CAD build for the part. Positions are in the model's coordinates, mm. A direction names the side the tool comes from. Coordinates: 2 decimals unless noted, no trailing zeros. Write each loop counter-clockwise with the first axis right and the second up, starting at its lowest first coordinate (ties: lowest second). Pieces come first, ordered by that corner, then holes. Notation, with made-up numbers: (-23, 41.25) - (25, 41.25) arc R26 ccw to (25, 61.25) - close; hole circle Ø6 at (79.25, -37.5). An arc over 180 degrees is marked (long way). One line per question, with ' | ' between items. Start each with the question number.
1. Band-saw the part on A-A, the plane z = -101. Write the cut outline in (x, y).
2. Two-plate mould, pull along X, no slides. Class faces 1 (the cylindrical face through (7.587, 34.168, 9.479)), 2 (the cylindrical face through (-28.4, -28.36, -60.49)), 3 (the cylindrical face through (-29.2, 29.81, 3.94)): +X half, -X half, draft (parallel to the pull), parting line (faces both ways), or undercut.
3. Band-saw the part on C-C, the plane y = -20.5. Write the cut outline in (x, z).
4. Flat gauge pins, fed straight in: P1, Ø8.5, axis at x = 31.82, y = 31.82, coming from the -Z side; P2, Ø7, axis at x = -35, z = -36, coming from the -Y side; P3, Ø2.5, axis at y = -33, z = -32, coming from the +X side; P4, Ø5.5, axis at x = 1, y = -0.5, coming from the +Z side. Where does each tip first touch, or does it go through?
5. Band-saw the part on B-B, the plane x = 0. Write the cut outline in (y, z).
6. Probe line 1 (Y direction, x = 0, z = 40); line 2 (Z direction, x = -12, y = -2); line 3 (Y direction, x = 31.5, z = -48.5). List the from-to ranges inside material, lowest first.
7. Band-saw the part on D-D, the plane x = -23. Write the cut outline in (y, z).
8. Which spindle directions (+Z, -Z, +X, -X, +Y, -Y) get a long thin tool onto all of the face, cutting with end or side? Do faces 4 (the flat face through (27.5, 35, -59)), 5 (the cylindrical face through (-28.4, 28.36, -60.49)), 6 (the flat face through (-35, -35, 0)), 7 (the flat face through (0, 12, 31)), 8 (the flat face through (0, 0, 33)). Say none if no direction does.
from build123d import *

# Parameters (mm, degrees)
SKETCH_1_W              = 80
SKETCH_1_H              = 80
EXTRUDE_1_DEPTH         = 8
FILLET_1_R              = 3
HOLE_WIZARD_6_6_6_6_1_D = 6.6
SKETCH_5_R              = 35
EXTRUDE_2_DEPTH         = 3
SKETCH_6_R              = 9.5
EXTRUDE_3_DEPTH         = 32
EXTRUDE_4_DEPTH         = 119.3
FILLET_2_R              = 3
FILLET_3_R              = 1
SKETCH_8_W              = 6
SKETCH_8_H              = 6
EXTRUDE_5_DEPTH         = 25
FILLET_4_R              = 0.5
SKETCH_9_R              = 2.5
CUT_EXTRUDE_1_DEPTH     = 10


with BuildPart() as part:
    # 草图1 → 凸台-拉伸1 (new body)
    with BuildSketch(Plane.XY):
        Rectangle(SKETCH_1_W, SKETCH_1_H)
    extrude(amount=EXTRUDE_1_DEPTH)

    # 圆角1
    fillet_1_edges = [part.edges().sort_by_distance(p)[0] for p in [
        (40, -40, 4),
        (-40, -40, 4),
        (-40, 40, 4),
        (40, 40, 4),
    ]]
    fillet(fillet_1_edges, radius=FILLET_1_R)

    # Ø6.6 (6.6) 直径孔1 (through all)
    with Locations(Plane.XY.offset(8)):
        with Locations((31.819805153, 31.819805153), (31.819805153, -31.819805153), (-31.819805153, -31.819805153), (-31.819805153, 31.819805153)):
            Hole(HOLE_WIZARD_6_6_6_6_1_D / 2)

    # 草图5 → 凸台-拉伸2 (add)
    with BuildSketch(Plane.XY.offset(8)):
        with Locations(Location((0, 0, 0), (0, 0, 180))):
            Circle(SKETCH_5_R)
    extrude(amount=EXTRUDE_2_DEPTH)

    # 草图6 → 凸台-拉伸3 (add)
    with BuildSketch(Plane.XY.offset(11)):
        Circle(SKETCH_6_R)
    extrude(amount=EXTRUDE_3_DEPTH)

    # 草图7 → 凸台-拉伸4 (add)
    with BuildSketch(Plane(origin=(0, 0, 0), x_dir=(-1, 0, 0), z_dir=(0, 0, -1))):
        Polygon((-27.5, 40), (27.5, 40), (27.5, 27.5), (40, 27.5), (40, -27.5), (27.5, -27.5), (27.5, -40), (-27.5, -40), (-27.5, -27.5), (-40, -27.5), (-40, 27.5), (-27.5, 27.5), align=None)
    extrude(amount=EXTRUDE_4_DEPTH)

    # 圆角2
    fillet_2_edges = [part.edges().sort_by_distance(p)[0] for p in [
        (27.5, -27.5, -59.65),
        (-27.5, -27.5, -59.65),
        (-27.5, 27.5, -59.65),
        (27.5, 27.5, -59.65),
    ]]
    fillet(fillet_2_edges, radius=FILLET_2_R)

    # 圆角3
    fillet_3_edges = [part.edges().sort_by_distance(p)[0] for p in [
        (40, -27.5, -59.65),
        (27.5, -40, -59.65),
        (-27.5, -40, -59.65),
        (-40, -27.5, -59.65),
        (-40, 27.5, -59.65),
        (-27.5, 40, -59.65),
        (27.5, 40, -59.65),
        (40, 27.5, -59.65),
    ]]
    fillet(fillet_3_edges, radius=FILLET_3_R)

    # 草图8 → 凸台-拉伸5 (add)
    with BuildSketch(Plane.XY.offset(43)):
        with Locations((0, 9)):
            Rectangle(SKETCH_8_W, SKETCH_8_H)
    extrude(amount=-EXTRUDE_5_DEPTH)

    # 圆角4
    fillet_4_edges = [part.edges().sort_by_distance(p)[0] for p in [
        (-5.556527693, -7.705517504, 43),
    ]]
    fillet(fillet_4_edges, radius=FILLET_4_R)

    # 草图9 → 切除-拉伸1 (cut)
    with BuildSketch(Plane.XY.offset(43)):
        Circle(SKETCH_9_R)
    extrude(amount=-CUT_EXTRUDE_1_DEPTH, mode=Mode.SUBTRACT)


solid = part.part
Filled in:
1) outline: (-40, -26.5) arc R1 ccw to (-39, -27.5) - (-30.5, -27.5) arc R3 cw to (-27.5, -30.5) - (-27.5, -39) arc R1 ccw to (-26.5, -40) - (26.5, -40) arc R1 ccw to (27.5, -39) - (27.5, -30.5) arc R3 cw to (30.5, -27.5) - (39, -27.5) arc R1 ccw to (40, -26.5) - (40, 26.5) arc R1 ccw to (39, 27.5) - (30.5, 27.5) arc R3 cw to (27.5, 30.5) - (27.5, 39) arc R1 ccw to (26.5, 40) - (-26.5, 40) arc R1 ccw to (-27.5, 39) - (-27.5, 30.5) arc R3 cw to (-30.5, 27.5) - (-39, 27.5) arc R1 ccw to (-40, 26.5) - close
2) face 1: parting line | face 2: -X half | face 3: undercut
3) outline: (-40, -119.3) - (40, -119.3) - (40, 8) - (28.37, 8) - (28.37, 11) - (-28.37, 11) - (-28.37, 8) - (-40, 8) - close
4) P1: stops at z = 0 | P2: stops at y = -27.5 | P3: stops at x = 27.5 | P4: stops at z = 43
5) outline: (-40, -119.3) - (40, -119.3) - (40, 8) - (35, 8) - (35, 11) - (9.5, 11) - (9.5, 18) - (12, 18) - (12, 43) - (2.5, 43) - (2.5, 33) - (-2.5, 33) - (-2.5, 43) - (-9, 43) arc R0.5 ccw to (-9.5, 42.5) - (-9.5, 11) - (-35, 11) - (-35, 8) - (-40, 8) - close
6) line 1: y = -9.5 to -2.5, 2.5 to 12 | line 2: z = -119.3 to 11 | line 3: y = -27.5 to 27.5
7) outline: (-40, -119.3) - (40, -119.3) - (40, 8) - (26.38, 8) - (26.38, 11) - (-26.38, 11) - (-26.38, 8) - (-40, 8) - close
8) face 4: -Z, +X, +Y | face 5: -Z, -X, +Y | face 6: -Z, -X, -Y | face 7: +Z, +X, -X, +Y | face 8: +Z
